Check sheet for the modelled part. Datum: model origin and axes. Units: mm. A direction names the side the tool comes from. Give positions to 0.01 mm unless a question says otherwise; leave off trailing zeros. Write each loop counter-clockwise with the first axis right and the second up, starting at its lowest first coordinate (ties: lowest second). Pieces come first, ordered by that corner, then holes. Notation, with made-up numbers: M 44.25,-16.5 L 74.25,-16.5 A18 cw 74.25,13.5 Z; hole C 85.25,-14 d2. An arc over 180 degrees is marked long. One line per item, written item: value. Start each with the question number.
from build123d import *

# Parameters (mm, degrees)
F0_R     = 4.5
F1_DEPTH = 1
F2_R     = 3
F3_DEPTH = 0.5
F4_R     = 2.05
F5_DEPTH = 1.5
F6_R     = 0.99999


# Not quite as in the source:
# - a fillet or chamfer is up to 0.001 mm smaller than in the source, because OpenCascade refuses the exact size


with BuildPart() as f1:
    # F0 (on Top) → F1 (new body)
    with BuildSketch(Plane.XY):
        Circle(F0_R)
    extrude(amount=F1_DEPTH)

    # F2 (on face) → F3 (join)
    with BuildSketch(Plane.XY.offset(1)):
        Circle(F2_R)
    extrude(amount=F3_DEPTH)

    # F4 (on face) → F5 (join)
    with BuildSketch(Plane.XY.offset(1.5)):
        Circle(F4_R)
    extrude(amount=F5_DEPTH)

    # F6 (radius 1 in the source; OpenCascade refuses exactly that, so slightly less here)
    f6_edges = [f1.edges().sort_by_distance(p)[0] for p in [
        (-4.5, 0, 0),
    ]]
    fillet(f6_edges, radius=F6_R)


solid = f1.part
1) Gauge pin test, flat ends, axial feed: pin 1 (2 mm diameter, centred on x = 1, y = -1, fed in from -Z); pin 2 (3 mm diameter, centred on x = 2, y = 3.5, fed in from +Z); pin 3 (1.5 mm diameter, centred on x = -2.5, z = 0.5, fed in from +Y). Record the tip position at first contact, or that the pin passes through.
2) Material ranges on L1, parallel to Z at x = -2.5, y = 0.25; L2, parallel to Z at x = 2.5, y = -2.25; L3, parallel to Y at x = 1, z = 1.8, recorded low to high. Write a range as from..to.
3) Cross-section at C-C (z = 2.4). Record the boundary of the cut face in (x, y).
4) Tool access check on faces 1 (the cylindrical face through (-3, 0.1, 1.2)), 2 (the flat face through (0, 0, 0)). Record the directions out of +Z, -Z, +X, -X, +Y, -Y that give a thin tool (end or side, any length) a straight path to the whole face; none if there is none.
Data:
1. pin 1: stops at z = 0
1. pin 2: stops at z = 1.5
1. pin 3: stops at y = 4.1
2. L1: z = 0..1.5
2. L2: z = 0..1
2. L3: y = -1.79..1.79
3. outline: C 0,0 d4.1
4. face 1: +Z
4. face 2: -Z, +X, -X, +Y, -Y
